from build123d import *

# Parameters (mm, degrees)
PCB_DIMENSIONS_W    = 47.716732244
PCB_DIMENSIONS_H    = 81.636732244
BOSS_EXTRUDE3_DEPTH = 1.5
SKETCH5_W           = 47.716732244
SKETCH5_H           = 81.636732244
SKETCH5_W_2         = 43.474091557
SKETCH5_H_2         = 73.394091557
BOSS_EXTRUDE5_DEPTH = 30
FILLET1_R           = 1
SKETCH9_W           = 1.93805105
SKETCH9_H           = 42
SKETCH9_W_2         = 1.938051049
BOSS_EXTRUDE6_DEPTH = 5
SKETCH14_W          = 15
SKETCH14_H          = 2.5
BOSS_EXTRUDE7_DEPTH = 3
SKETCH15_W          = 79.636732244
SKETCH15_H          = 3
BOSS_EXTRUDE8_DEPTH = 46
SKETCH17_W          = 39.522771214
SKETCH17_H          = 62.982276128
CUT_EXTRUDE1_DEPTH  = 3
CUT_EXTRUDE2_DEPTH  = 3
SKETCH19_W          = 11
SKETCH19_H          = 5
CUT_EXTRUDE3_DEPTH  = 10
FILLET2_R           = 1
SCALE1_SCALE        = 0.99


with BuildPart() as part:
    # PCB Dimensions → Boss-Extrude3 (new body)
    with BuildSketch(Plane(origin=(0, 0, 0), x_dir=(1, 0, 0), z_dir=(0, 1, 0))):
        with Locations((20.322832216, -37.282832216)):
            Rectangle(PCB_DIMENSIONS_W, PCB_DIMENSIONS_H)
    extrude(amount=BOSS_EXTRUDE3_DEPTH)

    # Sketch5 → Boss-Extrude5 (add)
    with BuildSketch(Plane(origin=(0, 1.5, 0), x_dir=(1, 0, 0), z_dir=(0, 1, 0))):
        with Locations((20.322832216, -37.282832216)):
            Rectangle(SKETCH5_W, SKETCH5_H)
        with Locations((20.322832217, -35.282832217)):
            Rectangle(SKETCH5_W_2, SKETCH5_H_2, mode=Mode.SUBTRACT)
    extrude(amount=BOSS_EXTRUDE5_DEPTH)

    # Fillet1
    fillet1_edges = [part.edges().sort_by_distance(p)[0] for p in [
        (42.059877995, 16.5, -1.414213562),
        (-1.414213562, 16.5, -1.414213562),
        (-1.414213562, 16.5, 71.979877995),
        (42.059877995, 16.5, 71.979877995),
        (44.181198338, 15.75, 78.101198338),
        (-3.535533906, 15.75, 78.101198338),
        (-3.535533906, 15.75, -3.535533906),
        (44.181198338, 15.75, -3.535533906),
    ]]
    fillet(fillet1_edges, radius=FILLET1_R)

    # Sketch9 → Boss-Extrude6 (add)
    with BuildSketch(Plane(origin=(0, 1.5, 0), x_dir=(1, 0, 0), z_dir=(0, 1, 0))):
        with Locations((-0.88911969, -49.979881394)):
            Rectangle(SKETCH9_W, SKETCH9_H)
        with Locations((41.534784122, -49.979881394)):
            Rectangle(SKETCH9_W_2, SKETCH9_H)
    extrude(amount=BOSS_EXTRUDE6_DEPTH)

    # Sketch14 → Boss-Extrude7 (add)
    with BuildSketch(Plane(origin=(0, 1.5, 0), x_dir=(1, 0, 0), z_dir=(0, 1, 0))):
        with Locations((6.085786438, -26.529881394)):
            Rectangle(SKETCH14_W, SKETCH14_H)
        with Locations((34.559877995, -26.529881394)):
            Rectangle(SKETCH14_W, SKETCH14_H)
    extrude(amount=BOSS_EXTRUDE7_DEPTH)

    # Sketch15 → Boss-Extrude8 (add)
    with BuildSketch(Plane(origin=(44.181198338, 0, 0), x_dir=(0, 0, -1), z_dir=(1, 0, 0))):
        with Locations((-37.282832216, 15.5)):
            Rectangle(SKETCH15_W, SKETCH15_H)
    extrude(amount=-BOSS_EXTRUDE8_DEPTH)

    # Sketch17 → Cut-Extrude1 (cut)
    with BuildSketch(Plane(origin=(0, 17, 0), x_dir=(1, 0, 0), z_dir=(0, 1, 0))):
        with Locations((20.322832216, -32.052584673)):
            Rectangle(SKETCH17_W, SKETCH17_H)
    extrude(amount=-CUT_EXTRUDE1_DEPTH, mode=Mode.SUBTRACT)

    # Sketch18 → Cut-Extrude2 (cut)
    with BuildSketch(Plane(origin=(0, 17, 0), x_dir=(1, 0, 0), z_dir=(0, 1, 0))):
        with BuildLine():
            Line((-1.414213562, -9.585786438), (28.585786438, -9.585786438))
            Line((28.585786438, -9.585786438), (28.585786438, 1.414213562))
            Line((28.585786438, 1.414213562), (-0.414213562, 1.414213562))
            ThreePointArc((-0.414213562, 1.414213562), (-1.121320344, 1.121320344), (-1.414213562, 0.414213562))
            Line((-1.414213562, 0.414213562), (-1.414213562, -9.585786438))
        make_face()
    extrude(amount=-CUT_EXTRUDE2_DEPTH, mode=Mode.SUBTRACT)

    # Sketch19 → Cut-Extrude3 (cut)
    with BuildSketch(Plane(origin=(44.181198338, 0, 0), x_dir=(0, 0, -1), z_dir=(1, 0, 0))):
        with Locations((-5.464466094, 21.15)):
            Rectangle(SKETCH19_W, SKETCH19_H)
    extrude(amount=-CUT_EXTRUDE3_DEPTH, mode=Mode.SUBTRACT)

    # Fillet2
    fillet2_edges = [part.edges().sort_by_distance(p)[0] for p in [
        (43.120538167, 23.65, -0.035533906),
        (43.120538167, 18.65, -0.035533906),
        (43.120538167, 18.65, 10.964466094),
        (43.120538167, 23.65, 10.964466094),
    ]]
    fillet(fillet2_edges, radius=FILLET2_R)


with BuildPart() as part_1:
    # Scale1: scaled about (20.311867002, 12.9416955, 45.018687776)
    add(part.part.scale(SCALE1_SCALE).moved(Location((0.20311867, 0.129416955, 0.450186878))))


solid = part_1.part
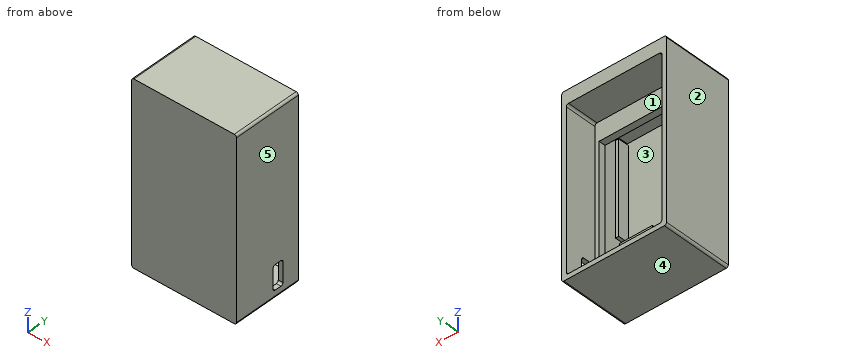
The model under review builds one solid part; all positions refer to its coordinate system, in mm. Face numbers are marked on the shaded views. A direction names the side the tool comes from. Round coordinates to 2 decimals unless told otherwise and drop trailing zeros. Order: outer loops, then holes, each group sorted by start corner. A loop starts at its lowest first (then second) coordinate and runs counter-clockwise, first axis right, second up. Notation, with made-up numbers: (-34.5, 60.25) -> (-6.5, 60.25) arc R10 ccw to (-6.5, 76.25) -> close; hole circle Ø10 at (86.25, 54.5). An arc over 180 degrees is marked (long way). Return JSON: item names as keys, results as strings.
1. Take a section at B-B (z = 58.5). Write out the cut boundary in (x, y).
Answer block:
{"outline": "(-3.3, 0.13) -> (43.94, 0.13) -> (43.94, 31.31) -> (41.84, 31.31) -> (41.84, 16.96) -> (39.89, 16.96) -> (39.89, 13.99) -> (41.84, 13.99) -> (41.84, 6.56) -> (40.36, 6.56) -> (40.36, 1.61) -> (0.28, 1.61) -> (0.28, 6.56) -> (-1.2, 6.56) -> (-1.2, 13.99) -> (0.76, 13.99) -> (0.76, 16.96) -> (-1.2, 16.96) -> (-1.2, 31.31) -> (-3.3, 31.31) -> close"}
2. Take a section at D-D (z = 24.5). Write out the cut boundary in (x, y), then the cut area to 3 significant figures.
Answer block:
{"outline": "(-3.3, 0.13) -> (43.94, 0.13) -> (43.94, 31.31) -> (41.84, 31.31) -> (41.84, 16.96) -> (39.89, 16.96) -> (39.89, 13.99) -> (41.84, 13.99) -> (41.84, 1.61) -> (-1.2, 1.61) -> (-1.2, 13.99) -> (0.76, 13.99) -> (0.76, 16.96) -> (-1.2, 16.96) -> (-1.2, 31.31) -> (-3.3, 31.31) -> close", "area": "207 mm²"}
3. For L1, parallel to Z at x = 5.5, y = 3; L2, parallel to Z at x = 40, y = 25; L3, parallel to X at y = 13.5, z = 67, list the stretches that pass through material, from the lowest coordinate up. Write a range as [from, to].
Answer block:
{"L1": "z = [-3.05, -0.95], [25.48, 27.95], [71.71, 77.77]", "L2": "z = [-3.05, -0.95], [71.71, 77.77]", "L3": "x = [-3.3, -1.2], [41.84, 43.94]"}
4. For the marked faces 1 and 2, list the 3-axis set-ups (+Z, -Z, +X, -X, +Y, -Y) from which the entire face can be reached by the end or side of a thin tool; tool diameter is ignored.
Answer block:
{"face 1": "+Y", "face 2": "+Z, -Z, -X, +Y, -Y"}
5. Take a section at A-A (y = 8). Write out the cut boundary in (x, z).
Answer block:
{"outline": "(-3.3, -2.06) arc R0.99 ccw to (-2.31, -3.05) -> (42.95, -3.05) arc R0.99 ccw to (43.94, -2.06) -> (43.94, 76.78) arc R0.99 ccw to (42.95, 77.77) -> (-2.31, 77.77) arc R0.99 ccw to (-3.3, 76.78) -> close; hole (-1.2, 0.04) arc R0.99 ccw to (-0.21, -0.95) -> (40.85, -0.95) arc R0.99 ccw to (41.84, 0.04) -> (41.84, 70.72) arc R0.99 ccw to (40.85, 71.71) -> (-0.21, 71.71) arc R0.99 ccw to (-1.2, 70.72) -> close"}
6. Insertion check: P1, Ø4, axis at x = 14.5, z = 46.5, coming from the +Y side. The pin has a flat end and moves straight along its axis. Give the tip position at first contact, or say it passes through.
Answer block:
{"P1": "stops at y = 1.61"}
7. Take a section at C-C (x = 7). Write out the cut boundary in (y, z).
Answer block:
{"outline": "(0.13, -3.05) -> (31.31, -3.05) -> (31.31, -0.95) -> (1.61, -0.95) -> (1.61, 25.48) -> (4.58, 25.48) -> (4.58, 27.95) -> (1.61, 27.95) -> (1.61, 71.71) -> (13.99, 71.71) -> (13.99, 63.36) -> (16.96, 63.36) -> (16.96, 71.71) -> (31.31, 71.71) -> (31.31, 77.77) -> (0.13, 77.77) -> close"}
8. The part is to be moulded in two halves that separate along Z. For the marked faces 3, 4 and 5, say which applies: +Z half, -Z half, draft (parallel to the pull), parting line (faces both ways), or undercut.
Answer block:
{"face 3": "undercut", "face 4": "-Z half", "face 5": "draft"}
